from build123d import *

# Parameters (mm, degrees)
SKETCH1_W           = 38.1
SKETCH1_H           = 82.55
BOSS_EXTRUDE1_DEPTH = 6.35
SKETCH2_W           = 5.08
SKETCH2_H           = 3.175
SKETCH2_W_2         = 3.175
SKETCH2_H_2         = 5.08
BOSS_EXTRUDE2_DEPTH = 6.35


with BuildPart() as part:
    # Sketch1 → Boss-Extrude1 (new body)
    with BuildSketch(Plane(origin=(0, 0, 0), x_dir=(1, 0, 0), z_dir=(0, 1, 0))):
        Rectangle(SKETCH1_W, SKETCH1_H)
    extrude(amount=BOSS_EXTRUDE1_DEPTH)

    # Sketch2 → Boss-Extrude2 (add)
    with BuildSketch(Plane(origin=(0, 0, 0), x_dir=(-1, 0, 0), z_dir=(0, -1, 0))):
        with Locations((-11.43, 42.8625)):
            Rectangle(SKETCH2_W, SKETCH2_H)
        with Locations((20.6375, 35.56)):
            Rectangle(SKETCH2_W_2, SKETCH2_H_2)
        with Locations((-1.27, 42.8625)):
            Rectangle(SKETCH2_W, SKETCH2_H)
        with Locations((8.89, 42.8625)):
            Rectangle(SKETCH2_W, SKETCH2_H)
        with Locations((20.6375, 25.4)):
            Rectangle(SKETCH2_W_2, SKETCH2_H_2)
        with Locations((20.6375, 15.24)):
            Rectangle(SKETCH2_W_2, SKETCH2_H_2)
        with Locations((20.6375, 5.08)):
            Rectangle(SKETCH2_W_2, SKETCH2_H_2)
        with Locations((20.6375, -5.08)):
            Rectangle(SKETCH2_W_2, SKETCH2_H_2)
        with Locations((20.6375, -15.24)):
            Rectangle(SKETCH2_W_2, SKETCH2_H_2)
        with Locations((20.6375, -25.4)):
            Rectangle(SKETCH2_W_2, SKETCH2_H_2)
        with Locations((20.6375, -35.56)):
            Rectangle(SKETCH2_W_2, SKETCH2_H_2)
        with Locations((8.89, -42.8625)):
            Rectangle(SKETCH2_W, SKETCH2_H)
        with Locations((-1.27, -42.8625)):
            Rectangle(SKETCH2_W, SKETCH2_H)
        with Locations((-11.43, -42.8625)):
            Rectangle(SKETCH2_W, SKETCH2_H)
    extrude(amount=-BOSS_EXTRUDE2_DEPTH)


solid = part.part
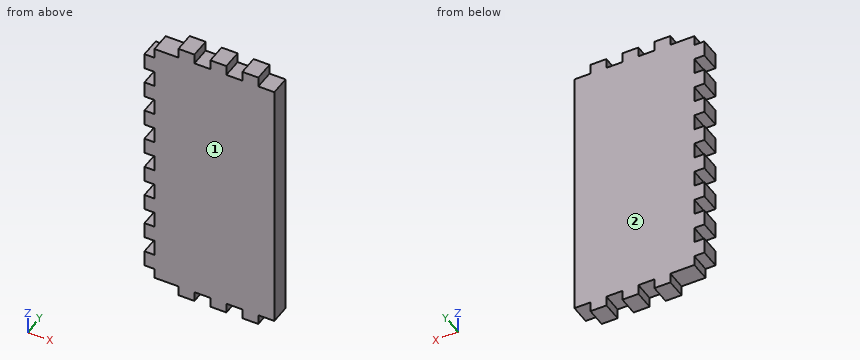
Could you check a few things on this model? Use its own coordinates, in mm. Face numbers are marked on the shaded views. Coordinates: 2 decimals unless noted, no trailing zeros. Loops run counter-clockwise (first coordinate to the right, second up) from the corner with the lowest first, then second, coordinate; pieces in that order, holes last.
1. We'd pull the mould along Y, two halves only. Please class the marked faces 1 and 2: released by +Y, released by -Y, zero draft, split by the parting line, or undercut.
2. For P1, Ø2.5, axis at y = 3, z = -43.5, coming from the -X side; P2, Ø2.5, axis at x = -20.5, y = 2, coming from the -Z side; P3, Ø1, axis at x = -21, y = 1.5, coming from the +Z side, each with a flat end and sliding along its axis, tell me the tip position at first contact or that it passes through.
3. I need wall thicknesses on L1, parallel to Z at x = -2, y = 5.25 (3 decimals); L2, parallel to X at y = 5.75, z = 31.5. Which ranges of each line are inside material? Lowest first, please.
4. Imagine slicing it at A-A (x = 5). Please give me the cut outline in (y, z) (3 decimals).
5. Imagine slicing it at B-B (z = 29.5). Please give me the cut outline in (x, y), and give its area (3 significant figures).
Computed values:
1. face 1: released by -Y
1. face 2: released by +Y
2. P1: stops at x = -11.43
2. P2: stops at z = -38.1
2. P3: stops at z = 38.1
3. L1: z = -41.275 to 41.275
3. L2: x = -19.05 to 19.05
4. outline: (0, -41.275) - (6.35, -41.275) - (6.35, 41.275) - (0, 41.275) - close
5. outline: (-19.05, 0) - (19.05, 0) - (19.05, 6.35) - (-19.05, 6.35) - close
5. area: 242 mm2
